Autodesk Inventor part; units mm, degrees
ref_plane "YZ Plane" through (0, 0, 0) normal (1, 0, 0) x (0, 1, 0)
ref_plane "XZ Plane" through (0, 0, 0) normal (0, 1, 0) x (-1, 0, 0)
ref_plane "XY Plane" through (0, 0, 0) normal (0, 0, 1) x (1, 0, 0)
sketch "Sketch1" plane through (0, 0, 0) normal (0, 0, 1) x (1, 0, 0)
  line L0 (-25, 65.19) -> (25, 65.19)
  line L1 (65.19, 25) -> (65.19, -25)
  line L2 (25, -65.19) -> (-25, -65.19)
  line L3 (-65.19, -25) -> (-65.19, 25)
  line L4 (-50.6308, 50.6308) -> (50.6308, -50.6308) construction
  line L5 (50, 50) -> (-50, -50) construction
  line L6 (-40, 40) -> (-50.6308, 50.6308) construction
  line L7 (-25, 65.19) -> (-25, 55.19)
  line L8 (-25, 55.19) -> (-35, 55.19)
  line L9 (-55.19, 35) -> (-55.19, 25)
  line L10 (-55.19, 25) -> (-65.19, 25)
  circle A0 centre (0, 0) radius 26
  line L11 (0, 28.0827) -> (0, 0)
  line L12 (0, 0) -> (17.6422, 0)
  line L13 (25, 65.19) -> (25, 55.19)
  line L14 (25, 55.19) -> (35, 55.19)
  line L15 (55.19, 35) -> (55.19, 25)
  line L16 (55.19, 25) -> (65.19, 25)
  line L17 (-25, -65.19) -> (-25, -55.19)
  line L18 (-25, -55.19) -> (-35, -55.19)
  line L19 (-55.19, -35) -> (-55.19, -25)
  line L20 (-55.19, -25) -> (-65.19, -25)
  line L21 (25, -65.19) -> (25, -55.19)
  line L22 (25, -55.19) -> (35, -55.19)
  line L23 (55.19, -35) -> (55.19, -25)
  line L24 (55.19, -25) -> (65.19, -25)
  line L25 (-35, 55.19) -> (-55.19, 35)
  line L26 (35, 55.19) -> (55.19, 35)
  line L27 (55.19, -35) -> (35, -55.19)
  line L28 (-35, -55.19) -> (-55.19, -35)
  point P0 (-45.3154, 45.3154)
  point P1 (-55.19, 55.19)
  point P2 (55.19, 55.19)
  point P3 (-55.19, -55.19)
  point P4 (55.19, -55.19)
  dimension "d9" = 130.38
  dimension "d19" = 10
  dimension "d20" = 52
  dimension "d40" = 130.38
  dimension "d45" = 10
  dimension "d58" = 50
  dimension "d59" = 50
  dimension "d60" = 20.19
  dimension "d61" = 20.19
  dimension "d62" = 20.19
  dimension "d63" = 20.19
  dimension "d64" = 20.19
  dimension "d65" = 20.19
  dimension "d66" = 20.19
  dimension "d67" = 20.19
  dimension "d79" = 10
extrude "Extrusion1" add sketch "Sketch1" along normal blind 10
sketch "Sketch3" plane through (0, 0, 10) normal (0, 0, 1) x (1, 0, 0)
  line L0 (25, 65.19) -> (-25, 65.19)
  line L1 (25, 65.19) -> (-25, 65.19)
  line L2 (-25, 65.19) -> (-25, 85)
  line L3 (-25, 85) -> (25, 85)
  line L4 (25, 85) -> (25, 65.19)
  line L5 (-25, 65.19) -> (-25, 55.19)
  circle A0 centre (-20, 80) radius 2.1
  line L6 (0, 0) -> (0, 7.5781)
  circle A1 centre (20, 80) radius 2.1
  circle A2 centre (-80, -20) radius 2.1
  circle A3 centre (-80, 20) radius 2.1
  circle A4 centre (20, -80) radius 2.1
  circle A5 centre (-20, -80) radius 2.1
  circle A6 centre (80, 20) radius 2.1
  circle A7 centre (80, -20) radius 2.1
  line L7 (25, 55.19) -> (25, 65.19)
  line L8 (-65.19, 25) -> (-65.19, -25)
  line L9 (-85, 25) -> (-65.19, 25)
  line L10 (-85, -25) -> (-85, 25)
  line L11 (-65.19, -25) -> (-85, -25)
  line L12 (-25, -65.19) -> (25, -65.19)
  line L13 (-25, -85) -> (-25, -65.19)
  line L14 (25, -85) -> (-25, -85)
  line L15 (25, -65.19) -> (25, -85)
  line L16 (65.19, -25) -> (65.19, 25)
  line L17 (85, -25) -> (65.19, -25)
  line L18 (85, 25) -> (85, -25)
  line L19 (65.19, 25) -> (85, 25)
  point P0 (-25, 60.19)
  point P1 (-25, 75.095)
  point P2 (-75.095, -25)
  point P3 (25, -75.095)
  point P4 (75.095, 25)
  dimension "d31" = 4.2
  dimension "d35" = 360
  dimension "d43" = 360
  dimension "d49" = 5
  dimension "d50" = 40
  dimension "d51" = 5
  dimension "d80" = 170
extrude "Extrusion3" add sketch "Sketch3" against normal up to surface (10 mm away)
sketch "Sketch5" plane through (0, 0, 0) normal (0, 0, -1) x (-1, 0, 0)
  circle A0 centre (0, 0) radius 26
  circle A1 centre (0, 0) radius 18.5
  dimension "d55" = 37
extrude "Extrusion5" add sketch "Sketch5" against normal blind 2
sketch "Sketch6" plane through (-35, 55.19, 0) normal (0, 1, 0) x (1, 0, 0)
  circle A0 centre (5, -5) radius 2.9
  line L0 (10, -10) -> (0, -10)
  line L1 (10, -10) -> (10, 0)
  point P0 (35, 0)
  dimension "d68" = 5
  dimension "d69" = 5
  dimension "d70" = 5.8
extrude "Extrusion6" cut sketch "Sketch6" against normal blind 10
mirror "Mirror1" about plane through (0, 0, 0) normal (1, 0, 0) of "Extrusion6"
pattern_circular "Circular Pattern2" count 4 over 360 about axis through (0, 0, 0) along (0, 0, 1) of "Extrusion6", "Mirror1"
equation "\"d9\" = d40"
equation "\"d59\" = d58"
properties part number "gearbox_base" material "PMMA Plastic"
Check sheet for the modelled part. Datum: model origin and axes. Units: mm. A direction names the side the tool comes from. Coordinates: 2 decimals unless noted, no trailing zeros. Loops run counter-clockwise (first coordinate to the right, second up) from the corner with the lowest first, then second, coordinate; pieces in that order, holes last. Notation, with made-up numbers: (-29.75, 37) -> (-19.75, 37) arc R19 cw to (-19.75, 51) -> close; hole circle Ø1 at (14, 63). An arc over 180 degrees is marked (long way). Answer in a Markdown table with one row per item.
1. Sectioned sample at D-D, the plane y = 50.5. Record the boundary of the cut face in (x, z).
Check values:
| item | result |
|---|---|
| outline | (-39.69, 0) -> (39.69, 0) -> (39.69, 10) -> (-39.69, 10) -> close; hole circle Ø5.8 at (-30, 5); hole circle Ø5.8 at (30, 5) |
2. Sectioned sample at C-C, the plane x = 4. Record the boundary of the cut face in (y, z), then the cut area to 3 significant figures.
Check values:
| item | result |
|---|---|
| outline | (-85, 0) -> (-18.06, 0) -> (-18.06, 2) -> (-25.69, 2) -> (-25.69, 10) -> (-85, 10) -> close; (18.06, 0) -> (85, 0) -> (85, 10) -> (25.69, 10) -> (25.69, 2) -> (18.06, 2) -> close |
| area | 1,220 mm2 |
3. Go/stop test with flat-tipped pins: pin 1 (4 mm diameter, centred on x = 61.5, z = 7.5, fed in from +Y); pin 2 (1 mm diameter, centred on y = 65, z = 4.5, fed in from -X); pin 3 (3 mm diameter, centred on x = -66.5, z = 2.5, fed in from -Y). Record where each tip stops, or that it passes through.
Check values:
| item | result |
|---|---|
| pin 1 | stops at y = 25 |
| pin 2 | stops at x = -25 |
| pin 3 | stops at y = -25 |
4. Access from +Z, -Z, +X, -X, +Y, -Y to the whole of each face (thin tool, end or side, straight path). Record for faces 1 (the face through (-70, -25, 5)), 2 (the face through (25, 70, 5)), 3 (the face through (27.234, 50.26, 5.871)).
Check values:
| item | result |
|---|---|
| face 1 | +Z, -Z, -X, -Y |
| face 2 | +Z, -Z, +X, +Y |
| face 3 | +Y |
5. Sectioned sample at A-A, the plane y = -80. Record the boundary of the cut face in (x, z), then the cut area to 3 significant figures.
Check values:
| item | result |
|---|---|
| outline | (-25, 0) -> (-22.1, 0) -> (-22.1, 10) -> (-25, 10) -> close; (-17.9, 0) -> (17.9, 0) -> (17.9, 10) -> (-17.9, 10) -> close; (22.1, 0) -> (25, 0) -> (25, 10) -> (22.1, 10) -> close |
| area | 416 mm2 |
6. Release check for a two-part mould opening along Y. For faces 4 (the face through (-50.26, -27.234, 4.129)), 5 (the face through (-30, -45.19, 5)), 6 (the face through (-85, 0, 5)) record: released by +Y, released by -Y, zero draft, split by the parting line, or undercut.
Check values:
| item | result |
|---|---|
| face 4 | undercut |
| face 5 | released by -Y |
| face 6 | zero draft |
7. Material ranges on line 1 along X through (y, z) = (-48.5, 5); line 2 along Y through (x, z) = (0, 6.5); line 3 along Y through (x, z) = (-19, 7.5), recorded low to high. Write a range as [from, to].
Check values:
| item | result |
|---|---|
| line 1 | x = [-41.69, -32.9], [-27.1, 27.1], [32.9, 41.69] |
| line 2 | y = [-85, -26], [26, 85] |
| line 3 | y = [-85, -81.85], [-78.15, -17.75], [17.75, 78.15], [81.85, 85] |
